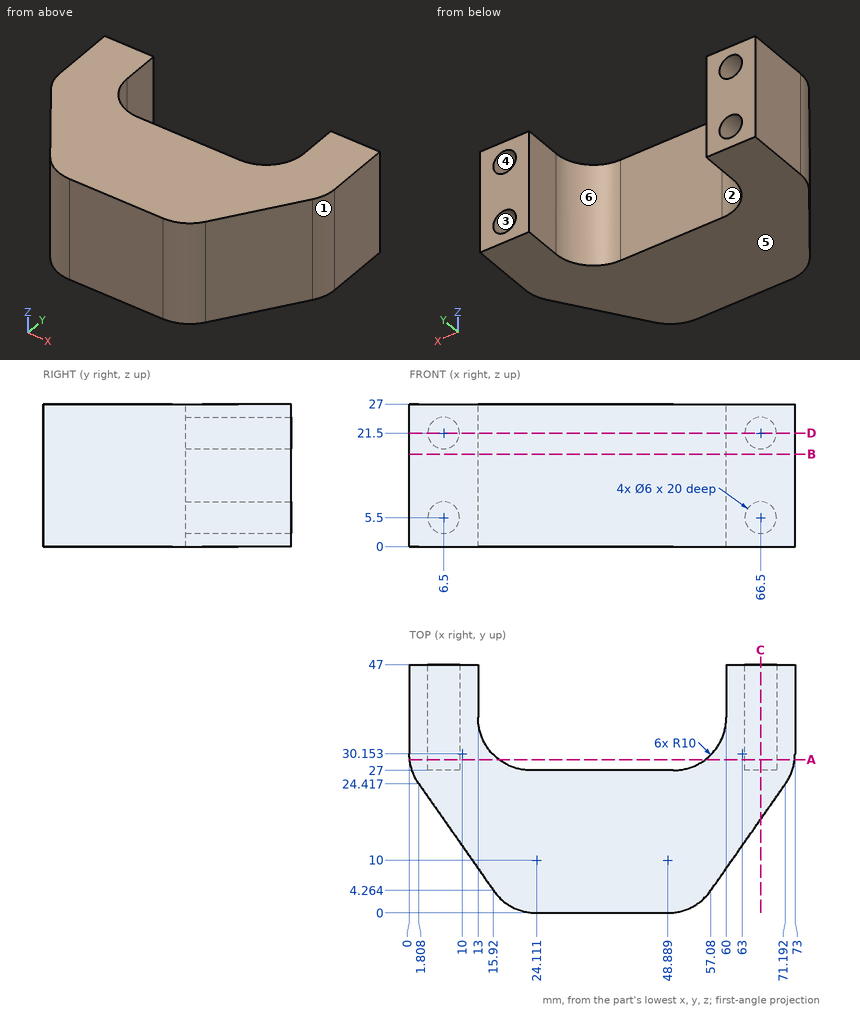
Job drawing, mm, ordinate dimensions from the low corner. One solid piece. A direction names the side the tool comes from. Coordinates: 2 decimals unless noted, no trailing zeros. Order: outer loops, then holes, each group sorted by start corner. A loop starts at its lowest first (then second) coordinate and runs counter-clockwise, first axis right, second up. Notation, with made-up numbers: (-6.5, 48) -> (7.5, 48) arc R16 ccw to (7.5, 52) -> close; hole circle Ø8 at (81.5, -40). An arc over 180 degrees is marked (long way). Put each result on its own line as item: value. Start each with the question number.
(1) Which spindle directions (+Z, -Z, +X, -X, +Y, -Y) get a long thin tool onto all of the face, cutting with end or side? Do the marked faces 1, 2 and 3. Say none if no direction does.
(2) Band-saw the part on C-C (x = 66.5). Give the cut face in (y, z).
(3) Probe line 1 along X through (y, z) = (38.5, 11.75); line 2 along X through (y, z) = (43, 3.5) (1 decimal); line 3 along X through (y, z) = (33, 5) (1 decimal). List the from-to ranges inside material, lowest first. Write a range as [from, to].
(4) Mould opens along Z. For the marked faces 4, 5 and 6 say: pulls with the +Z half, pulls with the -Z half, needs draft (parallel to the pull), parting line crosses it, or undercut.
(5) Band-saw the part on B-B (z = 17.5). Give the cut face in (x, y) (1 decimal).
(6) Pin check, flat tips, straight feed: pin 1 Ø2 at (x, y) = (38, 28.5) entering from +Z; pin 2 Ø9.5 at (x, z) = (6.5, 21.5) entering from -Y (1 decimal); pin 3 Ø8 at (x, z) = (66.5, 21.5) entering from -Y (1 decimal); pin 4 Ø3.5 at (x, z) = (66.5, 5.5) entering from -Y. Stop position of each tip, or through.
(7) Band-saw the part on D-D (z = 21.5). Give the cut face in (x, y) (1 decimal), then the cut area to 3 significant figures.
(8) Band-saw the part on A-A (y = 29). Give the cut face in (x, z).
Determined:
1. face 1: +Z, -Z, +X, -Y
1. face 2: +Z, -Z, +Y
1. face 3: +Y
2. outline: (17.72, 0) -> (47, 0) -> (47, 2.5) -> (27, 2.5) -> (27, 8.5) -> (47, 8.5) -> (47, 18.5) -> (27, 18.5) -> (27, 24.5) -> (47, 24.5) -> (47, 27) -> (17.72, 27) -> close
3. line 1: x = [0, 13], [60, 73]
3. line 2: x = [0, 4.3], [8.7, 13], [60, 64.3], [68.7, 73]
3. line 3: x = [0, 3.5], [9.5, 13.8], [59.2, 63.5], [69.5, 73]
4. face 4: undercut
4. face 5: pulls with the -Z half
4. face 6: needs draft
5. outline: (0, 30.2) arc R10 ccw to (1.8, 24.4) -> (15.9, 4.3) arc R10 ccw to (24.1, 0) -> (48.9, 0) arc R10 ccw to (57.1, 4.3) -> (71.2, 24.4) arc R10 ccw to (73, 30.2) -> (73, 47) -> (60, 47) -> (60, 37) arc R10 cw to (50, 27) -> (23, 27) arc R10 cw to (13, 37) -> (13, 47) -> (0, 47) -> close
6. pin 1: passes through
6. pin 2: stops at y = 10.9
6. pin 3: stops at y = 12
6. pin 4: stops at y = 15.22
7. outline: (0, 30.2) arc R10 ccw to (1.8, 24.4) -> (15.9, 4.3) arc R10 ccw to (24.1, 0) -> (48.9, 0) arc R10 ccw to (57.1, 4.3) -> (71.2, 24.4) arc R10 ccw to (73, 30.2) -> (73, 47) -> (69.5, 47) -> (69.5, 27) -> (63.5, 27) -> (63.5, 47) -> (60, 47) -> (60, 37) arc R10 cw to (50, 27) -> (23, 27) arc R10 cw to (13, 37) -> (13, 47) -> (9.5, 47) -> (9.5, 27) -> (3.5, 27) -> (3.5, 47) -> (0, 47) -> close
7. area: 1,770 mm²
8. outline: (0.07, 0) -> (17, 0) -> (17, 27) -> (0.07, 27) -> close; (56, 0) -> (72.93, 0) -> (72.93, 27) -> (56, 27) -> close; hole circle Ø6 at (6.5, 5.5); hole circle Ø6 at (6.5, 21.5); hole circle Ø6 at (66.5, 5.5); hole circle Ø6 at (66.5, 21.5)
